```python
from build123d import *

# Parameters (mm, degrees)
F0_W     = 20
F0_H     = 21
F0_H_2   = 9
F1_DEPTH = 25


with BuildPart() as f1:
    # F0 (on Front) → F1 (new body)
    with BuildSketch(Plane.XZ):
        with Locations((10, 19.5)):
            Rectangle(F0_W, F0_H)
        Polygon((20, 9), (20, 0), (30, 0), (40, 9.348061), (40, 19.348061), (30, 19.348061), (30, 40), (0, 40), (0, 30), (20, 30), align=None)
        with Locations((10, 4.5)):
            Rectangle(F0_W, F0_H_2)
    extrude(amount=F1_DEPTH)


solid = f1.part
```
Here's how the part is built. I have some questions about the finished solid (model axes, mm). A direction names the side the tool comes from. Give positions to 0.01 mm unless a question says otherwise; leave off trailing zeros. Order: outer loops, then holes, each group sorted by start corner. A loop starts at its lowest first (then second) coordinate and runs counter-clockwise, first axis right, second up. Notation, with made-up numbers: M 63.25,-35.5 L 107.25,-35.5 A18 cw 107.25,-10.5 Z; hole C 34.5,56 d5. An arc over 180 degrees is marked long. Use a Markdown table: item, result. Add a question column.
1. I need wall thicknesses on probe 1 along X at (y, z) = (-20.75, 27); probe 2 along X at (y, z) = (-9.5, 4.5). Which ranges of each line are inside material? Lowest first, please. Write a range as from..to.
2. Suppose I cut it at C-C (x = 33). List the corners of the cut face in (y, z) for me, and give its area (3 significant figures).
3. On a 3-axis mill with a long thin cutter (end or side, diameter ignored), from which of +Z, -Z, +X, -X, +Y, -Y can I reach the whole of each face in a straight line? I mean faces 1 (the flat face through (15, 0, 20)), 2 (the flat face through (35, -12, 19.348)). Say none if no direction works.
4. Suppose I cut it at B-B (z = 33.5). List the corners of the cut face in (x, y) for me.
5. For pin 1 Ø4 at (x, y) = (34, -14.5) entering from -Z; pin 2 Ø8 at (y, z) = (-22, 30.5) entering from -X; pin 3 Ø10.5 at (y, z) = (-14.5, 33.5) entering from +X; pin 4 Ø3 at (x, y) = (34, -9) entering from +Z, each with a flat end and sliding along its axis, tell me the tip position at first contact or that it passes through.
6. Suppose I cut it at A-A (y = -21.75). List the corners of the cut face in (x, z) for me, and give its area (3 significant figures).
Results list:
| question | item | result |
|---|---|---|
| 1 | probe 1 | x = 0..30 |
| 1 | probe 2 | x = 0..34.81 |
| 2 | outline | M -25,2.8 L 0,2.8 L 0,19.35 L -25,19.35 Z |
| 2 | area | 414 mm² |
| 3 | face 1 | +Z, -Z, +X, -X, +Y |
| 3 | face 2 | +Z, +X, +Y, -Y |
| 4 | outline | M 0,-25 L 30,-25 L 30,0 L 0,0 Z |
| 5 | pin 1 | stops at z = 1.87 |
| 5 | pin 2 | stops at x = 0 |
| 5 | pin 3 | stops at x = 30 |
| 5 | pin 4 | stops at z = 19.35 |
| 6 | outline | M 0,0 L 30,0 L 40,9.35 L 40,19.35 L 30,19.35 L 30,40 L 0,40 Z |
| 6 | area | 1,350 mm² |
